Could you check a few things on this model? Use its own coordinates, in mm. A direction names the side the tool comes from. Give positions to 0.01 mm unless a question says otherwise; leave off trailing zeros. Loops run counter-clockwise (first coordinate to the right, second up) from the corner with the lowest first, then second, coordinate; pieces in that order, holes last. Notation, with made-up numbers: M 68,5.5 L 87,5.5 A5 ccw 87,12.5 Z; hole C -23.5,14.25 d6. An arc over 180 degrees is marked long. Answer in a Markdown table with one row per item. Add a question column.
1. I need wall thicknesses on line 1 along X through (y, z) = (-1.25, 6.35); line 2 along Z through (x, y) = (571.5, -5); line 3 along Y through (x, z) = (116, 13.5). Which ranges of each line are inside material? Lowest first, please. Write a range as from..to.
2. If we section it at B-B on y = 11.75: List the corners of the cut face in (x, z) for me.
3. If we section it at C-C on x = 174: List the corners of the cut face in (y, z) for me, then the cut area to 3 significant figures.
4. Thinking about a two-plate mould opening in Z: for faces 3 (the flat face through (301, 9, 0)), 4 (the flat face through (609.6, -2, 1)), 5 (the cylindrical face through (16.983, -3.219, 3.619)), which applies, released by +Z, released by -Z, zero draft, split by the parting line, or undercut?
5. Which directions (+Z, -Z, +X, -X, +Y, -Y) give clear straight access to the entire face, cutting with the end or side of a thin tool? Please do faces 1 (the flat face through (301, 0, 10)), 2 (the flat face through (301, -6.35, 6)).
6. I'm going to push flat-ended pins straight in: pin 1 Ø4 at (x, y) = (110.5, 13) entering from +Z; pin 2 Ø1.5 at (x, z) = (343, 5) entering from +Y. Where does each tip first touch, or does it pass through?
7. If we section it at A-A on x = 12.7: List the corners of the cut face in (y, z) for me.
```python
from build123d import *

# Parameters (mm, degrees)
BOSS_EXTRUDE1_DEPTH = 609.6
SKETCH2_R           = 5.08
SKETCH2_R_2         = 3.175
SKETCH2_R_3         = 3.556
CUT_EXTRUDE1_DEPTH  = 914.4


with BuildPart() as part:
    # Sketch1 → Boss-Extrude1 (new body)
    with BuildSketch(Plane(origin=(0, 0, 0), x_dir=(0, 0, -1), z_dir=(1, 0, 0))):
        Polygon((0, 0), (0, 19.05), (6.35, 19.05), (6.35, -6.35), (-19.05, -6.35), (-19.05, 0), align=None)
    extrude(amount=BOSS_EXTRUDE1_DEPTH)

    # Sketch2 → Cut-Extrude1 (cut)
    with BuildSketch(Plane.XZ.offset(6.35)):
        with Locations(Location((12.7, 6.35, 0), (0, 0, 270))):
            Circle(SKETCH2_R)
        with Locations(Location((62.357, 6.35, 0), (0, 0, 270))):
            Circle(SKETCH2_R_2)
        with Locations(Location((596.9, 6.35, 0), (0, 0, 270))):
            Circle(SKETCH2_R_3)
        with Locations(Location((571.5, 6.35, 0), (0, 0, 270))):
            Circle(SKETCH2_R_3)
    extrude(amount=-CUT_EXTRUDE1_DEPTH, mode=Mode.SUBTRACT)


solid = part.part
```
Results:
| question | item | result |
|---|---|---|
| 1 | line 1 | 0..7.62, 17.78..59.18, 65.53..567.94, 575.06..593.34, 600.46..609.6 |
| 1 | line 2 | -6.35..2.79, 9.91..19.05 |
| 1 | line 3 | -6.35..0 |
| 2 | outline | M 0,-6.35 L 609.6,-6.35 L 609.6,0 L 0,0 Z |
| 3 | outline | M -6.35,-6.35 L 19.05,-6.35 L 19.05,0 L 0,0 L 0,19.05 L -6.35,19.05 Z |
| 3 | area | 282 mm2 |
| 4 | face 3 | released by +Z |
| 4 | face 4 | zero draft |
| 4 | face 5 | undercut |
| 5 | face 1 | +Z, +X, -X, +Y |
| 5 | face 2 | +Z, -Z, +X, -X, -Y |
| 6 | pin 1 | z = 0 |
| 6 | pin 2 | y = 0 |
| 7 | outline | M -6.35,-6.35 L 19.05,-6.35 L 19.05,0 L 0,0 L 0,1.27 L -6.35,1.27 Z; M -6.35,11.43 L 0,11.43 L 0,19.05 L -6.35,19.05 Z |
